Could you check a few things on this model? Use its own coordinates, in mm. A direction names the side the tool comes from. Give positions to 0.01 mm unless a question says otherwise; leave off trailing zeros. Write each loop counter-clockwise with the first axis right and the second up, starting at its lowest first coordinate (ties: lowest second). Pieces come first, ordered by that corner, then holes. Notation, with made-up numbers: (18.25, -2) -> (22.25, -2) arc R17 ccw to (22.25, 2) -> close; hole circle Ø8 at (-1.5, -24.75). An arc over 180 degrees is marked (long way). One line per question, with ' | ' between items.
from build123d import *

# Parameters (mm, degrees)
BOSS_EXTRUDE1_DEPTH = 10
BOSS_EXTRUDE2_DEPTH = 910
FILLET1_R           = 20


with BuildPart() as part:
    # Sketch1 → Boss-Extrude1 (new body)
    with BuildSketch(Plane.XY):
        Polygon((0, 405), (285, 250), (285, 0), (0, 0), align=None)
    boss_extrude1 = extrude(amount=-BOSS_EXTRUDE1_DEPTH)

    # Sketch2 → Boss-Extrude2 (add)
    with BuildSketch(Plane.XY):
        Polygon((10, 0), (285, 0), (285, 10), (10, 10), (10, 399.561403509), (0, 405), (0, 10), (0, 0), align=None)
    extrude(amount=-BOSS_EXTRUDE2_DEPTH)

    # Mirror1: Boss-Extrude1 across plane
    add(boss_extrude1.mirror(Plane(origin=(0, 0, -460), x_dir=(1, 0, 0), z_dir=(0, 0, -1))))

    # Fillet1
    fillet1_edges = [part.edges().sort_by_distance(p)[0] for p in [
        (10, 204.780701754, -10),
        (10, 204.780701754, -910),
    ]]
    fillet(fillet1_edges, radius=FILLET1_R)


solid = part.part
Q1. If we mould it in two halves opening along Z, with no side actions, what happens to faces 3 (the flat face through (144, 160, 0)), 4 (the flat face through (0, 200, -466)), 5 (the flat face through (159, 160, -10))? For each: +Z half, -Z half, draft (parallel to the pull), parting line (faces both ways), or undercut.
Answer below:
face 3: +Z half | face 4: draft | face 5: undercut
Q2. Imagine slicing it at B-B on x = 166. Please give me the cut outline in (y, z).
Answer below:
outline: (0, -920) -> (314.72, -920) -> (314.72, -910) -> (10, -910) -> (10, -10) -> (314.72, -10) -> (314.72, 0) -> (0, 0) -> close
Q3. Imagine slicing it at D-D on y = 167. Please give me the cut outline in (x, z), and give its area (3 significant figures).
Answer below:
outline: (0, -920) -> (285, -920) -> (285, -910) -> (30, -910) arc R20 cw to (10, -890) -> (10, -30) arc R20 cw to (30, -10) -> (285, -10) -> (285, 0) -> (0, 0) -> close | area: 14,900 mm^2
Q4. Imagine slicing it at A-A on y = 312. Please give me the cut outline in (x, z).
Answer below:
outline: (0, -920) -> (171, -920) -> (171, -910) -> (30, -910) arc R20 cw to (10, -890) -> (10, -30) arc R20 cw to (30, -10) -> (171, -10) -> (171, 0) -> (0, 0) -> close
Q5. If I drill on line 1 along Z through (x, y) = (161.5, 128); line 2 along X through (y, z) = (217, -532); line 3 along Z through (x, y) = (20.5, 18), over which ranges is the centre line in solid material (lowest first)?
Answer below:
line 1: z = -920 to -910, -10 to 0 | line 2: x = 0 to 10 | line 3: z = -920 to -907.6, -12.4 to 0
Q6. Imagine slicing it at C-C on z = -670.5. Please give me the cut outline in (x, y), and give its area (3 significant figures).
Answer below:
outline: (0, 0) -> (285, 0) -> (285, 10) -> (10, 10) -> (10, 399.56) -> (0, 405) -> close | area: 6,770 mm^2
Q7. On a 3-axis mill with a long thin cutter (end or side, diameter ignored), from which of +Z, -Z, +X, -X, +Y, -Y can I reach the whole of each face in a straight line? I mean faces 1 (the flat face through (144, 160, -920)), 2 (the cylindrical face through (16.014, 202.054, -15.703)). Say none if no direction works.
Answer below:
face 1: -Z, +X, -X, +Y, -Y | face 2: +X, +Y
Q8. Will this pin go through, and if not, where does the flat tip stop? pin 1 (1 mm diameter, centred on x = 150, z = -242, fed in from +Y).
Answer below:
pin 1: stops at y = 10
